Check sheet for the modelled part. Datum: model origin and axes. Units: mm. A direction names the side the tool comes from. Coordinates: 2 decimals unless noted, no trailing zeros. Order: outer loops, then holes, each group sorted by start corner. A loop starts at its lowest first (then second) coordinate and runs counter-clockwise, first axis right, second up.
1. Cross-section at A-A (x = 85). Enter the section's corners in (y, z).
2. Thickness scan on line 1 (Y direction, x = 85, z = 395.3); line 2 (Y direction, x = 77, z = 394.75); line 3 (X direction, y = -36, z = 394.6). Record the ranges inside material, lowest first.
3. Gauge pin test, flat ends, axial feed: pin 1 Ø1.5 at (y, z) = (-13, 396) entering from -X; pin 2 Ø1.1 at (y, z) = (-31, 396) entering from +X; pin 3 Ø12 at (x, y) = (89.5, -31) entering from +Z. Record the tip position at first contact, or that the pin passes through.
4. Draft check along X on faces 4 (the flat face through (85, -10, 394)), 5 (the flat face through (100.89, -18.45, 395.48)), 6 (the cylindrical face through (72.4, 0.1, 395.5)). Enter one of: released by +X, released by -X, zero draft, split by the parting line, or undercut.
5. Cross-section at D-D (x = 93.5). Enter the section's corners in (y, z), then the cut area to 3 significant figures.
6. Cross-section at B-B (y = 0). Enter the section's corners in (x, z).
7. Set-up check for faces 1 (the cylindrical face through (84.8, -41.7, 395.5)), 2 (the flat face through (75, -31, 395)), 3 (the flat face through (95, -31, 395)): record each of +Z, -Z, +X, -X, +Y, -Y from which the full face is reachable in a straight line by a thin tool's end or side.
8. Cross-section at C-C (z = 395.7). Enter the section's corners in (x, y), then the cut area to 3 significant figures.
```python
from build123d import *

# Parameters (mm, degrees)
SKETCH058_R     = 6
SKETCH058_R_2   = 2.6
PAD019_DEPTH    = 3
FILLET011_R     = 10
CHAMFER018_SIZE = 3


with BuildPart() as part:
    # Sketch058 → Pad019 (new body)
    with BuildSketch(Plane.XY):
        with BuildLine():
            Line((-20, -10), (-20, 10))
            Line((-20, 10), (20, 10))
            Line((20, 10), (20, -10))
            Line((20, -10), (20, -15))
            Line((15.358186, -18.894945), (20, -15))
            ThreePointArc((15.358186, -18.894945), (11.405383, -24.046337), (10, -30.385611))
            Line((10, -30.385611), (10, -31.7))
            ThreePointArc((-10, -31.7), (0, -41.7), (10, -31.7))
            Line((-10, -30.385611), (-10, -31.7))
            ThreePointArc((-10, -30.385611), (-11.405383, -24.046337), (-15.358186, -18.894945))
            Line((-15.358186, -18.894945), (-20, -15))
            Line((-20, -10), (-20, -15))
        make_face()
        with Locations((0, -31.7)):
            Circle(SKETCH058_R, mode=Mode.SUBTRACT)
        with Locations((-10, 0)):
            Circle(SKETCH058_R_2, mode=Mode.SUBTRACT)
        with Locations((10, 0)):
            Circle(SKETCH058_R_2, mode=Mode.SUBTRACT)
    extrude(amount=PAD019_DEPTH)

    # Fillet011
    fillet011_edges = [part.edges().sort_by_distance(p)[0] for p in [
        (-20, -15, 1.5),
        (20, -15, 1.5),
    ]]
    fillet(fillet011_edges, radius=FILLET011_R)

    # Chamfer018
    chamfer018_edges = [part.edges().sort_by_distance(p)[0] for p in [
        (-20, 10, 1.5),
        (20, 10, 1.5),
    ]]
    chamfer(chamfer018_edges, length=CHAMFER018_SIZE)


with BuildPart() as part_1:
    # Body011 placement: moved
    add(part.part.moved(Location((85, 0, 394))))


solid = part_1.part
```
Data:
1. outline: (-41.7, 394) - (-37.7, 394) - (-37.7, 397) - (-41.7, 397) - close; (-25.7, 394) - (10, 394) - (10, 397) - (-25.7, 397) - close
2. line 1: y = -41.7 to -37.7, -25.7 to 10
2. line 2: y = -37.7 to -1.66, 1.66 to 10
2. line 3: x = 75.97 to 80.82, 89.18 to 94.03
3. pin 1: stops at x = 65.18
3. pin 2: stops at x = 95
3. pin 3: stops at z = 397
4. face 4: zero draft
4. face 5: released by +X
4. face 6: undercut
5. outline: (-36.97, 394) - (-2.12, 394) - (-2.12, 397) - (-36.97, 397) - close; (2.12, 394) - (10, 394) - (10, 397) - (2.12, 397) - close
5. area: 128 mm2
6. outline: (65, 394) - (72.4, 394) - (72.4, 397) - (65, 397) - close; (77.6, 394) - (92.4, 394) - (92.4, 397) - (77.6, 397) - close; (97.6, 394) - (105, 394) - (105, 397) - (97.6, 397) - close
7. face 1: +Z, -Z, -Y
7. face 2: +Z, -Z, -X, -Y
7. face 3: +Z, -Z, +X, -Y
8. outline: (65, -10.34) arc R10 ccw to (68.57, -18) - (69.64, -18.89) arc R15 cw to (75, -30.39) - (75, -31.7) arc R10 ccw to (95, -31.7) - (95, -30.39) arc R15 cw to (100.36, -18.89) - (101.43, -18) arc R10 ccw to (105, -10.34) - (105, 7) - (102, 10) - (68, 10) - (65, 7) - close; hole circle Ø5.2 at (75, 0); hole circle Ø12 at (85, -31.7); hole circle Ø5.2 at (95, 0)
8. area: 1,420 mm2
